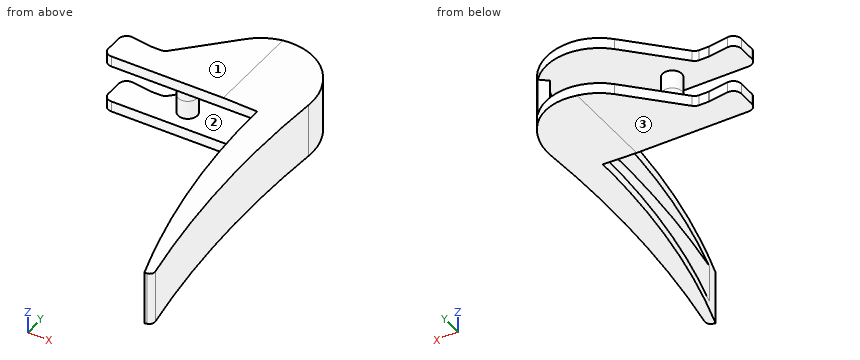
from build123d import *

# Parameters (mm, degrees)
BOSS_EXTRUDE1_DEPTH             = 5.5
BOSS_EXTRUDE1_DEPTH_BACK        = 5.5
SHELL4_START                    = -3.5
SHELL4_DEPTH                    = 7
CUT_EXTRUDE1_DEPTH              = 55.655740778
CUT_EXTRUDE1_DEPTH_BACK         = 55.655740778
SKETCH2_W                       = 69.221398806
SKETCH2_H                       = 30.475534722
BOSS_EXTRUDE2_REACH             = 56.656
SKETCH3_R                       = 1.8
BOSS_EXTRUDE2_DIRECTION_2_REACH = 56.656
FILLET1_R                       = 1.5
FILLET2_R                       = 1


# Read off the part's stored shape, not the designer's step: Shell4
with BuildPart() as part:
    # Sketch1 → Boss-Extrude1 (new, two sides: drawn at the far end of the back side and taken through both)
    with BuildSketch(Plane.XY.offset(-BOSS_EXTRUDE1_DEPTH_BACK)):
        with BuildLine():
            Line((0, 0), (-29, 0))
            Line((-29, 0), (-29, 6.4))
            Line((-29, 6.4), (-23.5, 5.6))
            Line((-23.5, 5.6), (-21, 5.6))
            Line((-21, 5.6), (-11.679922193, 15.24784279))
            ThreePointArc((-11.679922193, 15.24784279), (-4.185109089, 18.295419669), (3.11160179, 14.8))
            ThreePointArc((3.11160179, 14.8), (5.40105274, 10.720543521), (5.956739646, 6.07567938))
            ThreePointArc((5.956739646, 6.07567938), (5.643205462, -19.921417521), (8.704665249, -45.739527733))
            Line((8.704665249, -45.739527733), (7.227453619, -46))
            ThreePointArc((7.227453619, -46), (1.817879019, -23.282161013), (0, 0))
        make_face()
    extrude(amount=BOSS_EXTRUDE1_DEPTH + BOSS_EXTRUDE1_DEPTH_BACK)

    # Shell4 outline → Shell4 (cut)
    with BuildSketch(Plane.XY.offset(SHELL4_START)):
        with BuildLine():
            Line((1.591733374, 13.5), (3.11160179, 14.8))
            ThreePointArc((3.11160179, 14.8), (-4.185109088, 18.295419669), (-11.679922193, 15.24784279))
            Line((-11.679922193, 15.24784279), (-21, 5.6))
            Line((-21, 5.6), (-23.5, 5.6))
            Line((-23.5, 5.6), (-29, 6.4))
            Line((-29, 6.4), (-29, 0))
            Line((-29, 0), (0, 0))
            ThreePointArc((0, 0), (1.520272061, -21.301887027), (6.050271879, -42.171978539))
            ThreePointArc((6.050271879, -42.171978539), (3.550168012, -18.033934193), (3.962681588, 6.229732817))
            ThreePointArc((3.962681588, 6.229732817), (3.499609166, 10.100452934), (1.591733374, 13.5))
        make_face()
    extrude(amount=SHELL4_DEPTH, mode=Mode.SUBTRACT)

    # Sketch2 → Cut-Extrude1 (cut, two sides: drawn at the far end of the back side and taken through both)
    with BuildSketch(Plane(origin=(0, 0, 0), x_dir=(1, 0, 0), z_dir=(0, 1, 0)).offset(-CUT_EXTRUDE1_DEPTH_BACK)):
        Rectangle(SKETCH2_W, SKETCH2_H)
        Polygon((-29, 6.25), (8.704665249, 5), (8.704665249, -5), (-29, -6.25), align=None, mode=Mode.SUBTRACT)
    extrude(amount=CUT_EXTRUDE1_DEPTH + CUT_EXTRUDE1_DEPTH_BACK, mode=Mode.SUBTRACT)

    # Boss-Extrude2: up to this face of the body (flat: up to its plane)
    boss_extrude2_end = Plane(part.part.faces().sort_by_distance((-7.261638812, 3.224340324, 3.5))[0])
    # Sketch3 → Boss-Extrude2 (add, up to the picked face)
    with BuildSketch(Plane.XY, mode=Mode.PRIVATE) as boss_extrude2_sk1:
        with Locations(Location((-15.555262484, 4, 0), (0, 0, 180))):
            Circle(SKETCH3_R)
    boss_extrude2_tool1 = split(extrude(boss_extrude2_sk1.sketch, amount=BOSS_EXTRUDE2_REACH, mode=Mode.PRIVATE), bisect_by=boss_extrude2_end, keep=Keep.BOTH, mode=Mode.PRIVATE)
    add(boss_extrude2_tool1.solids().sort_by(Axis((-15.555262, 4, 0), (0, 0, 1)))[0])

    # Boss-Extrude2 direction 2: up to this face of the body (flat: up to its plane)
    boss_extrude2_direction_2_end = Plane(part.part.faces().sort_by_distance((-7.261638812, 3.224340324, -3.5))[0])
    # Sketch3 → Boss-Extrude2 direction 2 (add, up to the picked face)
    with BuildSketch(Plane.XY, mode=Mode.PRIVATE) as boss_extrude2_direction_2_sk1:
        with Locations(Location((-15.555262484, 4, 0), (0, 0, 180))):
            Circle(SKETCH3_R)
    boss_extrude2_direction_2_tool1 = split(extrude(boss_extrude2_direction_2_sk1.sketch, amount=-BOSS_EXTRUDE2_DIRECTION_2_REACH, mode=Mode.PRIVATE), bisect_by=boss_extrude2_direction_2_end, keep=Keep.BOTH, mode=Mode.PRIVATE)
    add(boss_extrude2_direction_2_tool1.solids().sort_by(Axis((-15.555262, 4, 0), (0, 0, -1)))[0])

    # Fillet1
    fillet1_edges = [part.edges().sort_by_distance(p)[0] for p in [
        (-29, 0, -4.5),
        (-29, 6.4, -4.5),
        (-23.5, 5.6, -4.5),
        (-21, 5.6, -4.5),
        (-21, 5.6, 4.5),
        (-23.5, 5.6, 4.5),
        (-29, 6.4, 4.5),
        (-29, 0, 4.5),
    ]]
    fillet(fillet1_edges, radius=FILLET1_R)

    # Fillet2
    fillet2_edges = [part.edges().sort_by_distance(p)[0] for p in [
        (8.704665249, -45.739527733, 0),
    ]]
    fillet(fillet2_edges, radius=FILLET2_R)


solid = part.part
CAD build for the part. Positions are in the model's coordinates, mm. Face numbers are marked on the shaded views. Coordinates: 2 decimals unless noted, no trailing zeros. Loops run counter-clockwise (first coordinate to the right, second up) from the corner with the lowest first, then second, coordinate; pieces in that order, holes last. Notation, with made-up numbers: (11, -7) - (40, -7) arc R25 cw to (40, 9) - close; hole circle Ø6 at (29, 32). An arc over 180 degrees is marked (long way). Write item = value, one per line. Start each with the question number.
Q1. Cut at B-B, the plane y = 4. List the corners of the cut face in (x, z).
Q2. Drill centre lines: L1, parallel to Z at x = 0.5, y = 15.5; L2, parallel to X at y = -9, z = -0.75; L3, parallel to Z at x = 2.5, y = 3.5. Where is each one in solid material? Low to high.
Q3. Cut at A-A, the plane y = -15. List the corners of the cut face in (x, z).
Q4. Cut at C-C, the plane x = -14.5. List the corners of the cut face in (y, z), then the cut area to 3 significant figures.
Q5. Flat gauge pins, fed straight in: pin 1 Ø1.6 at (x, z) = (-16, -4.5) entering from -Y; pin 2 Ø5 at (x, z) = (1.5, -4) entering from +Y; pin 3 Ø0.5 at (x, z) = (-22, -5) entering from +Y; pin 4 Ø10 at (x, y) = (-18.5, -1) entering from -Z. Where does each tip first touch, or does it go through?
Q6. Cut at D-D, the plane y = -23.5. List the corners of the cut face in (x, z).
Q7. Pull direction Z, two halves, no side cores. Call the marked faces 1, 2 and 3: pulls with the +Z half, pulls with the -Z half, needs draft (parallel to the pull), parting line crosses it, or undercut.
Computed:
q1.outline = (-29, -5.5) - (-6.38, -5.5) - (5.81, -5.1) - (5.81, 5.1) - (-6.38, 5.5) - (-29, 5.5) - (-29, 3.5) - (-17.36, 3.5) - (-17.36, -3.5) - (-29, -3.5) - close; hole (-13.76, -3.5) - (3.8, -3.5) - (3.8, 3.5) - (-13.76, 3.5) - close
q2.L1 = -5.27 to -3.5, 3.5 to 5.27
q2.L2 = 3.36 to 5.36
q2.L3 = -5.21 to -3.5, 3.5 to 5.21
q3.outline = (0.75, -5.26) - (5.44, -5.11) - (5.44, 5.11) - (0.75, 5.26) - (0.75, 3.5) - (3.44, 3.5) - (3.44, -3.5) - (0.75, -3.5) - close
q4.outline = (0, -5.5) - (12.33, -5.5) - (12.33, -3.5) - (5.46, -3.5) - (5.46, 3.5) - (12.33, 3.5) - (12.33, 5.5) - (0, 5.5) - (0, 3.5) - (2.54, 3.5) - (2.54, -3.5) - (0, -3.5) - close
q4.area = 69.7 mm²
q5.pin_1 = 0
q5.pin_2 = 17.67
q5.pin_3 = 5.6
q5.pin_4 = -5.5
q6.outline = (1.85, -5.23) - (5.87, -5.09) - (5.87, 5.09) - (1.85, 5.23) - (1.85, 3.5) - (3.86, 3.5) - (3.86, -3.5) - (1.85, -3.5) - close
q7.face_1 = pulls with the +Z half
q7.face_2 = undercut
q7.face_3 = pulls with the -Z half
